CAD build for the part. Positions are in the model's coordinates, mm. Face numbers are marked on the shaded views. A direction names the side the tool comes from. Give positions to 0.01 mm unless a question says otherwise; leave off trailing zeros. Write each loop counter-clockwise with the first axis right and the second up, starting at its lowest first coordinate (ties: lowest second). Pieces come first, ordered by that corner, then holes. Notation, with made-up numbers: (83, -18.75) -> (95, -18.75) arc R27 cw to (95, 5.25) -> close; hole circle Ø6 at (68, 86). An arc over 180 degrees is marked (long way). Answer as a JSON object with one key per item and string values.
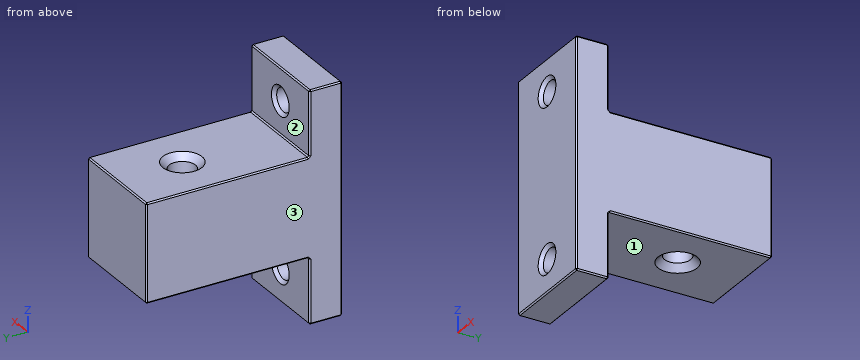
```python
from build123d import *

# Parameters (mm, degrees)
SKETCH1_W                      = 19.05
SKETCH1_H                      = 44.45
SKETCH1_H_2                    = 19.05
BOSS_EXTRUDE1_DEPTH            = 6.35
SKETCH1_3_W                    = 19.05
SKETCH1_3_H                    = 19.05
BOSS_EXTRUDE2_DEPTH            = 38.1
F_8_CLEARANCE_HOLE1_AT_2_COUNT = 2
F_8_CLEARANCE_HOLE1_AT_2_PITCH = 31.75
CHAMFER1_SIZE                  = 0.254


with BuildPart() as part:
    # Sketch1 → Boss-Extrude1 (new body)
    with BuildSketch(Plane(origin=(0, 0, 0), x_dir=(1, 0, 0), z_dir=(0, 1, 0))):
        Rectangle(SKETCH1_W, SKETCH1_H)
        Rectangle(SKETCH1_W, SKETCH1_H_2)
    extrude(amount=BOSS_EXTRUDE1_DEPTH)

    # Sketch1<3> → Boss-Extrude2 (add)
    with BuildSketch(Plane(origin=(0, 0, 0), x_dir=(1, 0, 0), z_dir=(0, 1, 0))):
        Rectangle(SKETCH1_3_W, SKETCH1_3_H)
    extrude(amount=BOSS_EXTRUDE2_DEPTH)

    # Sketch4 → 1/4-20 Tapped Hole1 (revolve, cut)
    with BuildSketch(Plane(origin=(0, 25.4, 9.525), x_dir=(0, -1, 0), z_dir=(1, 0, 0))):
        Polygon((0, 0), (0, 19.05), (3.81, 19.05), (2.5527, 17.7927), (2.5527, 1.2573), (3.81, 0), align=None)
    revolve(axis=Axis((0, 25.4, 15.875), (0, 0, -1)), mode=Mode.SUBTRACT)

    # Sketch8 → #8 Clearance Hole1 (revolve, cut)
    with BuildSketch(Plane(origin=(0, 6.35, -15.875), x_dir=(0, 0, 1), z_dir=(1, 0, 0))):
        Polygon((0, 0), (0, 6.35), (2.8829, 6.35), (2.2479, 5.715), (2.2479, 0.635), (2.8829, 0), align=None)
    f_8_clearance_hole1 = revolve(axis=Axis((0, 12.7, -15.875), (0, -1, 0)), mode=Mode.SUBTRACT)

    # #8 Clearance Hole1 at 2: #8 Clearance Hole1 ×2
    with Locations(*[(0, 0, i * F_8_CLEARANCE_HOLE1_AT_2_PITCH) for i in range(1, F_8_CLEARANCE_HOLE1_AT_2_COUNT)]):
        add(f_8_clearance_hole1, mode=Mode.SUBTRACT)

    # Chamfer1
    chamfer1_edges = [part.edges().sort_by_distance(p)[0] for p in [
        (0, 6.35, -22.225),
        (-9.525, 6.35, 15.875),
        (9.525, 6.35, -15.875),
        (-9.525, 6.35, -15.875),
        (0, 6.35, 22.225),
        (0, 6.35, 9.525),
        (9.525, 22.225, -9.525),
        (0, 6.35, -9.525),
        (0, 38.1, -9.525),
        (-9.525, 22.225, -9.525),
        (-9.525, 38.1, 0),
        (-9.525, 22.225, 9.525),
        (9.525, 22.225, 9.525),
        (0, 38.1, 9.525),
        (9.525, 38.1, 0),
        (9.525, 6.35, 15.875),
        (0, 0, 22.225),
        (-9.525, 0, 0),
        (0, 0, -22.225),
        (9.525, 0, 0),
        (9.525, 3.175, 22.225),
        (-9.525, 3.175, 22.225),
        (-9.525, 3.175, -22.225),
        (9.525, 3.175, -22.225),
    ]]
    chamfer(chamfer1_edges, length=CHAMFER1_SIZE)


solid = part.part
```
1) Wall check: probe 1 along Z at (x, y) = (0, 3.55) (3 decimals); probe 2 along Y at (x, z) = (-7, -19); probe 3 along Y at (x, z) = (0, 2.5). Give the ranges that are in metal, low to high.
Model answer:
{"probe 1": "z = -22.225 to -18.123, -13.627 to 13.627, 18.123 to 22.225", "probe 2": "y = 0 to 6.35", "probe 3": "y = 0 to 22.85, 27.95 to 38.1"}
2) Pin check, flat tips, straight feed: pin 1 (1.5 mm diameter, centred on x = 4.5, y = 24, fed in from -Z) (3 decimals); pin 2 (4 mm diameter, centred on x = 0, z = 16.5, fed in from +Y); pin 3 (1.5 mm diameter, centred on x = 5, y = 15.5, fed in from +Z) (3 decimals). Stop position of each tip, or through.
Model answer:
{"pin 1": "stops at z = -9.525", "pin 2": "stops at y = 6.09", "pin 3": "stops at z = 9.525"}
3) Slice it at C-C (x = -7.75). List the corners of the cut face in (y, z) (3 decimals), then the cut area to 3 significant figures.
Model answer:
{"outline": "(0, -21.971) -> (0.254, -22.225) -> (6.096, -22.225) -> (6.35, -21.971) -> (6.35, -9.779) -> (6.604, -9.525) -> (37.846, -9.525) -> (38.1, -9.271) -> (38.1, 9.271) -> (37.846, 9.525) -> (6.604, 9.525) -> (6.35, 9.779) -> (6.35, 21.971) -> (6.096, 22.225) -> (0.254, 22.225) -> (0, 21.971) -> close", "area": "887 mm2"}
4) Slice it at D-D (y = 12.5). List the corners of the cut face in (x, z) (3 decimals), then the cut area to 3 significant figures.
Model answer:
{"outline": "(-9.525, -9.271) -> (-9.271, -9.525) -> (9.271, -9.525) -> (9.525, -9.271) -> (9.525, 9.271) -> (9.271, 9.525) -> (-9.271, 9.525) -> (-9.525, 9.271) -> close", "area": "363 mm2"}
5) 3-axis set-ups, long thin cutter, end or side, ignore diameter. For the marked faces 1, 2 and 3: which of +Z, -Z, +X, -X, +Y, -Y reach the whole face in a straight line?
Model answer:
{"face 1": "-Z, +X, -X, +Y", "face 2": "+Z, +X, -X, +Y", "face 3": "+Z, -Z, -X, +Y, -Y"}
6) Slice it at B-B (y = 5). List the corners of the cut face in (x, z) (3 decimals), then the cut area to 3 significant figures.
Model answer:
{"outline": "(-9.525, -21.971) -> (-9.271, -22.225) -> (9.271, -22.225) -> (9.525, -21.971) -> (9.525, 21.971) -> (9.271, 22.225) -> (-9.271, 22.225) -> (-9.525, 21.971) -> close; hole circle Ø4.496 at (0, -15.875); hole circle Ø4.496 at (0, 15.875)", "area": "815 mm2"}
7) Slice it at A-A (y = 25.4). List the corners of the cut face in (x, z) (3 decimals), then the cut area to 3 significant figures.
Model answer:
{"outline": "(-9.525, -9.271) -> (-9.271, -9.525) -> (-3.81, -9.525) -> (-2.553, -8.268) -> (-2.553, 8.268) -> (-3.81, 9.525) -> (-9.271, 9.525) -> (-9.525, 9.271) -> close; (2.553, -8.268) -> (3.81, -9.525) -> (9.271, -9.525) -> (9.525, -9.271) -> (9.525, 9.271) -> (9.271, 9.525) -> (3.81, 9.525) -> (2.553, 8.268) -> close", "area": "262 mm2"}
